Input: part model. Units: mm. Frame: model coordinates. A direction names the side the tool comes from. Give positions to 0.01 mm unless a question says otherwise; leave off trailing zeros. Loops run counter-clockwise (first coordinate to the right, second up) from the corner with the lowest first, then second, coordinate; pieces in that order, holes last.
from build123d import *

# Parameters (mm, degrees)
SKETCH_2_R          = 4.2
EXTRUDE_1_DEPTH     = 25
FILLET_1_R          = 3
CUT_EXTRUDE_1_DEPTH = 25
SKETCH_4_W          = 2
SKETCH_4_H          = 9.772408651
SKETCH_4_H_2        = 10.02993421
CUT_EXTRUDE_2_DEPTH = 25
SKETCH_5_R          = 1.25
CUT_EXTRUDE_3_DEPTH = 35
SKETCH_6_R          = 1.7
CUT_EXTRUDE_4_DEPTH = 32


with BuildPart() as part:
    # 草图2 → 凸台-拉伸1 (new body)
    with BuildSketch(Plane(origin=(0, 0, 0), x_dir=(1, 0, 0), z_dir=(0, 1, 0))):
        Polygon((-10.5, 44.6), (-10.5, 34.8), (-1.5, 34.8), (-1.5, 39.7), (1.5, 39.7), (1.5, -36.1), (-1.5, -36.1), (-1.5, -31.2), (-10.5, -31.2), (-10.5, -41), (-13.5, -41), (-13.5, 44.6), align=None)
        with Locations(Location((-6, -23.2, 0), (0, 0, 270))):
            Circle(SKETCH_2_R, mode=Mode.SUBTRACT)
        with Locations(Location((-6, 26.8, 0), (0, 0, 270))):
            Circle(SKETCH_2_R, mode=Mode.SUBTRACT)
    extrude(amount=EXTRUDE_1_DEPTH)

    # 圆角1
    fillet_1_edges = [part.edges().sort_by_distance(p)[0] for p in [
        (1.5, 12.5, 36.1),
        (1.5, 12.5, -39.7),
        (-10.5, 12.5, -34.8),
        (-10.5, 12.5, 31.2),
        (-13.5, 12.5, -44.6),
        (-13.5, 12.5, 41),
    ]]
    fillet(fillet_1_edges, radius=FILLET_1_R - 0.0001)  # a hair under: the kernel refuses the full size

    # 草图3 → 切除-拉伸1 (cut)
    with BuildSketch(Plane(origin=(0, 25, 0), x_dir=(1, 0, 0), z_dir=(0, 1, 0))):
        with BuildLine():
            Line((-7.5, 18.8), (-4.5, 18.8))
            ThreePointArc((-4.5, 18.8), (-2.378679656, 17.921320344), (-1.5, 15.8))
            Line((-1.5, 15.8), (-1.5, -12.2))
            ThreePointArc((-1.5, -12.2), (-2.378679656, -14.321320344), (-4.5, -15.2))
            Line((-4.5, -15.2), (-7.5, -15.2))
            ThreePointArc((-7.5, -15.2), (-9.621320344, -14.321320344), (-10.5, -12.2))
            Line((-10.5, -12.2), (-10.5, 15.8))
            ThreePointArc((-10.5, 15.8), (-9.621320344, 17.921320344), (-7.5, 18.8))
        make_face()
    extrude(amount=-CUT_EXTRUDE_1_DEPTH, mode=Mode.SUBTRACT)

    # 草图4 → 切除-拉伸2 (cut)
    with BuildSketch(Plane(origin=(0, 25, 0), x_dir=(1, 0, 0), z_dir=(0, 1, 0))):
        with Locations((-6, -31.836216801)):
            Rectangle(SKETCH_4_W, SKETCH_4_H)
        with Locations((-6, 32.148208176)):
            Rectangle(SKETCH_4_W, SKETCH_4_H_2)
    extrude(amount=-CUT_EXTRUDE_2_DEPTH, mode=Mode.SUBTRACT)

    # 草图5 → 切除-拉伸3 (cut)
    with BuildSketch(Plane(origin=(1.5, 0, 0), x_dir=(0, 0, -1), z_dir=(1, 0, 0))):
        with Locations((-21.2, 15)):
            Circle(SKETCH_5_R)
        with Locations((24.8, 15)):
            Circle(SKETCH_5_R)
    extrude(amount=-CUT_EXTRUDE_3_DEPTH, mode=Mode.SUBTRACT)

    # 草图6 → 切除-拉伸4 (cut)
    with BuildSketch(Plane(origin=(1.5, 0, 0), x_dir=(0, 0, -1), z_dir=(1, 0, 0))):
        with Locations((26.8, 5)):
            Circle(SKETCH_6_R)
        with Locations((26.8, 20)):
            Circle(SKETCH_6_R)
        with Locations((-23.2, 5)):
            Circle(SKETCH_6_R)
        with Locations((-23.2, 20)):
            Circle(SKETCH_6_R)
    extrude(amount=-CUT_EXTRUDE_4_DEPTH, mode=Mode.SUBTRACT)


solid = part.part
(1) Pin query (flat end, axial travel): pin 1 Ø1.8 at (x, y) = (-3, 9) entering from +Z; pin 2 Ø8 at (x, y) = (-3.5, 16) entering from +Z; pin 3 Ø3.5 at (x, y) = (-5.5, 16.5) entering from -Z. Return the tip coordinate at first contact, or that it passes through.
Values follow:
pin 1: stops at z = 31.2
pin 2: stops at z = 36.1
pin 3: stops at z = -34.8
(2) Ray query, probe 1 along Y at (x, z) = (-10.6, -26.8); probe 2 along Z at (x, y) = (-6.25, 20.25); probe 3 along X at (y, z) = (16, -26.8). Return the intervals inside material, ascending.
Values follow:
probe 1: y = 0 to 3.3, 6.7 to 18.3, 21.7 to 25
probe 2: z = -22.61 to -18.8, 15.2 to 19.01
probe 3: x = -13.5 to -10.2, -1.8 to 1.5
(3) Cut plane A-A (z = -10). Return the cut outline in (x, y).
Values follow:
outline: (-13.5, 0) - (-10.5, 0) - (-10.5, 25) - (-13.5, 25) - close; (-1.5, 0) - (1.5, 0) - (1.5, 25) - (-1.5, 25) - close
(4) Cut plane B-B (z = 23.2). Return the cut outline in (x, y), and give its area (3 significant figures).
Values follow:
outline: (-13.5, 0) - (-10.2, 0) - (-10.2, 3.3) - (-13.5, 3.3) - close; (-13.5, 6.7) - (-10.2, 6.7) - (-10.2, 18.3) - (-13.5, 18.3) - close; (-13.5, 21.7) - (-10.2, 21.7) - (-10.2, 25) - (-13.5, 25) - close; (-1.8, 0) - (1.5, 0) - (1.5, 3.3) - (-1.8, 3.3) - close; (-1.8, 6.7) - (1.5, 6.7) - (1.5, 18.3) - (-1.8, 18.3) - close; (-1.8, 21.7) - (1.5, 21.7) - (1.5, 25) - (-1.8, 25) - close
area: 120 mm2
(5) Mould query, pull axis Y, two halves, no side actions, for faces 1 (the cylindrical face through (-11.64, 20.07, -25.1)), 2 (the flat face through (-1.5, 12, 34)). Classes: +Y half, -Y half, draft (parallel to the pull), parting line (faces both ways), or undercut.
Values follow:
face 1: undercut
face 2: draft
(6) Cut plane C-C (x = -6). Return the cut outline in (y, z), and give its area (3 significant figures).
Values follow:
outline: (0, -22.6) - (25, -22.6) - (25, -18.8) - (0, -18.8) - close; (0, 15.2) - (25, 15.2) - (25, 19) - (0, 19) - close
area: 190 mm2
(7) Reachability of faces 3 (the flat face through (-5, 13, -33)), 4 (the cylindrical face through (-11.58, 15.38, 20.01)), 5 (the flat face through (-6, 13, -18.8)) from +Z, -Z, +X, -X, +Y, -Y: full face, straight path, thin tool, end or side. Return the list, or none.
Values follow:
face 3: -Z, +Y, -Y
face 4: +X, -X
face 5: +Y, -Y
